```python
from build123d import *

# Parameters (mm, degrees)
BOSS_EXTRUDE1_DEPTH             = 4.763
M2_5_CLEARANCE_HOLE1_D          = 2.9
TAP_DRILL_FOR_M3X0_5_TAP1_D     = 2.5
TAP_DRILL_FOR_M3X0_5_TAP1_DEPTH = 4.763


with BuildPart() as part:
    # Sketch1 → Boss-Extrude1 (new body)
    with BuildSketch(Plane(origin=(0, 0, 0), x_dir=(1, 0, 0), z_dir=(0, 1, 0))):
        with BuildLine():
            Line((-61.5, 17.5), (-26.191601707, 17.5))
            ThreePointArc((-26.191601707, 17.5), (-22.273863607, 22.273863607), (-17.5, 26.191601707))
            Line((-17.5, 26.191601707), (-17.5, 61.5))
            Line((-17.5, 61.5), (17.5, 61.5))
            Line((17.5, 61.5), (17.5, 26.191601707))
            ThreePointArc((17.5, 26.191601707), (22.273863607, 22.273863607), (26.191601707, 17.5))
            Line((26.191601707, 17.5), (61.5, 17.5))
            Line((61.5, 17.5), (61.5, -17.5))
            Line((61.5, -17.5), (26.191601707, -17.5))
            ThreePointArc((26.191601707, -17.5), (22.273863607, -22.273863607), (17.5, -26.191601707))
            Line((17.5, -26.191601707), (17.5, -61.5))
            Line((17.5, -61.5), (-17.5, -61.5))
            Line((-17.5, -61.5), (-17.5, -26.191601707))
            ThreePointArc((-17.5, -26.191601707), (-22.273863607, -22.273863607), (-26.191601707, -17.5))
            Line((-26.191601707, -17.5), (-61.5, -17.5))
            Line((-61.5, -17.5), (-61.5, 17.5))
        make_face()
        with BuildLine():
            Line((-18.299951333, 4.863661227), (-28.657445997, 8.22916814))
            ThreePointArc((-28.657445997, 8.22916814), (-29.929968402, 8.100940268), (-30.69495913, 7.075979368))
            ThreePointArc((-30.69495913, 7.075979368), (-31.5, 0), (-30.69495913, -7.075979368))
            ThreePointArc((-30.69495913, -7.075979368), (-29.929968402, -8.100940268), (-28.657445997, -8.22916814))
            Line((-28.657445997, -8.22916814), (-18.299951333, -4.863661227))
            ThreePointArc((-18.299951333, -4.863661227), (-17.4289221, -4.170054209), (-17.227734354, -3.074925855))
            ThreePointArc((-17.227734354, -3.074925855), (-17.5, 0), (-17.227734354, 3.074925855))
            ThreePointArc((-17.227734354, 3.074925855), (-17.4289221, 4.170054209), (-18.299951333, 4.863661227))
        make_face(mode=Mode.SUBTRACT)
        with BuildLine():
            Line((-4.863661227, 18.299951333), (-8.22916814, 28.657445997))
            ThreePointArc((-8.22916814, 28.657445997), (-8.100940268, 29.929968402), (-7.075979368, 30.69495913))
            ThreePointArc((-7.075979368, 30.69495913), (0, 31.5), (7.075979368, 30.69495913))
            ThreePointArc((7.075979368, 30.69495913), (8.100940268, 29.929968402), (8.22916814, 28.657445997))
            Line((8.22916814, 28.657445997), (4.863661227, 18.299951333))
            ThreePointArc((4.863661227, 18.299951333), (4.170054209, 17.4289221), (3.074925855, 17.227734354))
            ThreePointArc((3.074925855, 17.227734354), (0, 17.5), (-3.074925855, 17.227734354))
            ThreePointArc((-3.074925855, 17.227734354), (-4.170054209, 17.4289221), (-4.863661227, 18.299951333))
        make_face(mode=Mode.SUBTRACT)
        with BuildLine():
            Line((18.299951333, 4.863661227), (28.657445997, 8.22916814))
            ThreePointArc((28.657445997, 8.22916814), (29.929968402, 8.100940268), (30.69495913, 7.075979368))
            ThreePointArc((30.69495913, 7.075979368), (31.5, 0), (30.69495913, -7.075979368))
            ThreePointArc((30.69495913, -7.075979368), (29.929968402, -8.100940268), (28.657445997, -8.22916814))
            Line((28.657445997, -8.22916814), (18.299951333, -4.863661227))
            ThreePointArc((18.299951333, -4.863661227), (17.4289221, -4.170054209), (17.227734354, -3.074925855))
            ThreePointArc((17.227734354, -3.074925855), (17.5, 0), (17.227734354, 3.074925855))
            ThreePointArc((17.227734354, 3.074925855), (17.4289221, 4.170054209), (18.299951333, 4.863661227))
        make_face(mode=Mode.SUBTRACT)
        with BuildLine():
            Line((4.863661227, -18.299951333), (8.22916814, -28.657445997))
            ThreePointArc((8.22916814, -28.657445997), (8.100940268, -29.929968402), (7.075979368, -30.69495913))
            ThreePointArc((7.075979368, -30.69495913), (0, -31.5), (-7.075979368, -30.69495913))
            ThreePointArc((-7.075979368, -30.69495913), (-8.100940268, -29.929968402), (-8.22916814, -28.657445997))
            Line((-8.22916814, -28.657445997), (-4.863661227, -18.299951333))
            ThreePointArc((-4.863661227, -18.299951333), (-4.170054209, -17.4289221), (-3.074925855, -17.227734354))
            ThreePointArc((-3.074925855, -17.227734354), (0, -17.5), (3.074925855, -17.227734354))
            ThreePointArc((3.074925855, -17.227734354), (4.170054209, -17.4289221), (4.863661227, -18.299951333))
        make_face(mode=Mode.SUBTRACT)
    extrude(amount=BOSS_EXTRUDE1_DEPTH)

    # M2.5 Clearance Hole1 (through all)
    with Locations(Plane(origin=(0, 4.763, 0), x_dir=(1, 0, 0), z_dir=(0, 1, 0))):
        with Locations((5.303300859, 5.303300859), (-5.303300859, 5.303300859), (-5.303300859, -5.303300859), (5.303300859, -5.303300859)):
            Hole(M2_5_CLEARANCE_HOLE1_D / 2)

    # Tap Drill for M3x0.5 Tap1
    with Locations(Plane(origin=(0, 4.763, 0), x_dir=(1, 0, 0), z_dir=(0, 1, 0))):
        with Locations((-56.7375, 14.65), (-30.954101707, 14.65), (-56.7375, -14.65), (30.954101707, 14.65), (56.5, 14.65), (-30.954101707, -14.65), (30.954101707, -14.65), (56.5, -14.65), (-14.65, 56.7375), (14.65, 56.7375), (-14.65, -56.7375), (14.65, -56.7375)):
            Hole(TAP_DRILL_FOR_M3X0_5_TAP1_D / 2, depth=TAP_DRILL_FOR_M3X0_5_TAP1_DEPTH)


solid = part.part
```
Geometry: final body of the model. Coordinates: model frame, mm. A direction names the side the tool comes from. Round coordinates to 2 decimals unless told otherwise and drop trailing zeros. Order: outer loops, then holes, each group sorted by start corner. A loop starts at its lowest first (then second) coordinate and runs counter-clockwise, first axis right, second up. Notation, with made-up numbers: (34.5, -13) -> (53.5, -13) arc R13 cw to (53.5, 10) -> close; hole circle Ø10 at (7, -23.75). An arc over 180 degrees is marked (long way). Use one line per item in the form item = value. Start each with the question number.
1. Cut plane B-B (x = 47.5). Return the cut outline in (y, z).
2. Cut plane A-A (x = 22.5). Return the cut outline in (y, z).
3. Reachability of faces 1 (the face through (-17.5, 2, 44)), 2 (the face through (1, 0, -1)), 3 (the face through (-17.5, 2, -44)), 4 (the face through (0.1, 2.3, 31.5)) from +Z, -Z, +X, -X, +Y, -Y: full face, straight path, thin tool, end or side. Return the list, or none.
4. Draft query along X for faces 5 (the face through (-22.21, 2.35, 22.34)), 6 (the face through (1, 4.763, -1)), 7 (the face through (17.5, 2, 44)), 8 (the face through (-6.643, 2.348, -4.748)). Return one class per face: pulls with the +X half, pulls with the -X half, needs draft (parallel to the pull), parting line crosses it, or undercut.
5. Pin query (flat end, axial travel): pin 1 Ø2.5 at (x, y) = (-47.5, 1.5) entering from -Z. Return the tip coordinate at first contact, or that it passes through.
6. Cut plane C-C (z = -47). Return the cut outline in (x, y), then the cut area to 3 significant figures.
7. Line query: probe 1 along Z at (x, y) = (14.65, 3.75); probe 2 along Z at (x, y) = (-0.5, 4.5); probe 3 along X at (y, z) = (0.65, 3). Output: solid intervals per line, ascending.
8. Cut plane D-D (y = 0.75). Count the separate pieces of the cut face and the enclosed holes in it, then the cut area to 3 significant figures.
Solution:
q1.outline = (0, -17.5) -> (4.76, -17.5) -> (4.76, 17.5) -> (0, 17.5) -> close
q2.outline = (0, -22.05) -> (4.76, -22.05) -> (4.76, -6.23) -> (0, -6.23) -> close; (0, 6.23) -> (4.76, 6.23) -> (4.76, 22.05) -> (0, 22.05) -> close
q3.face_1 = +Z, -X, +Y, -Y
q3.face_2 = +Z, -Z, +X, -X, -Y
q3.face_3 = -Z, -X, +Y, -Y
q3.face_4 = +Y, -Y
q4.face_5 = pulls with the -X half
q4.face_6 = needs draft
q4.face_7 = pulls with the +X half
q4.face_8 = undercut
q5.pin_1 = -17.5
q6.outline = (-17.5, 0) -> (17.5, 0) -> (17.5, 4.76) -> (-17.5, 4.76) -> close
q6.area = 167 mm^2
q7.probe_1 = -61.5 to -57.99, -55.49 to 55.49, 57.99 to 61.5
q7.probe_2 = -61.5 to -31.5, -17.49 to 17.49, 31.5 to 61.5
q7.probe_3 = -61.5 to -31.36, -17.24 to 17.24, 31.36 to 61.5
q8.separate_pieces = 1
q8.enclosed_holes = 20
q8.area = 6,730 mm^2
